Can you work these out from the model? Positions are in its coordinate system, mm. A direction names the side the tool comes from. Give positions to 0.01 mm unless a question says otherwise; leave off trailing zeros. Loops run counter-clockwise (first coordinate to the right, second up) from the corner with the lowest first, then second, coordinate; pieces in that order, holes last. Notation, with made-up numbers: (73, 67) - (81, 67) arc R32 cw to (81, 94) - close; hole circle Ø7 at (27, -12). An arc over 180 degrees is marked (long way). Answer in a Markdown table with one row per item.
from build123d import *

# Parameters (mm, degrees)
REVOLVE1_ANGLE      = 180
BOSS_EXTRUDE2_DEPTH = 8
REVOLVE2_ANGLE      = 180
SWEEP1_PROFILE_R    = 0.5
SWEEP2_PROFILE_R    = 0.5


with BuildPart() as part:
    # Sketch3 → Revolve1 (revolve)
    with BuildSketch(Plane(origin=(0, 0, 0), x_dir=(0, 0, -1), z_dir=(1, 0, 0))):
        with BuildLine():
            Line((-32, 4), (-2, 4))
            ThreePointArc((-2, 4), (-1.5, 3.5), (-1, 4))
            Line((-1, 4), (0, 4))
            Line((0, 4), (0, 0))
            Line((0, 0), (-32, 0))
            Line((-32, 0), (-32, 4))
        make_face()
    revolve(axis=Axis((0, 0, 32.603933811), (0, 0, -1)), revolution_arc=REVOLVE1_ANGLE)

    # Sketch4 → Boss-Extrude2 (add)
    with BuildSketch(Plane.ZY):
        with BuildLine():
            Line((0, 4), (0, -4))
            Line((0, -4), (1, -4))
            ThreePointArc((1, -4), (1.5, -3.5), (2, -4))
            Line((2, -4), (32, -4))
            Line((32, -4), (32, 4))
            Line((32, 4), (2, 4))
            ThreePointArc((2, 4), (1.5, 3.5), (1, 4))
            Line((1, 4), (0, 4))
        make_face()
    extrude(amount=BOSS_EXTRUDE2_DEPTH)

    # Sketch5 → Revolve2 (revolve)
    with BuildSketch(Plane.ZY.offset(8)):
        with BuildLine():
            Line((0, 0), (0, 4))
            Line((0, 4), (1, 4))
            ThreePointArc((1, 4), (1.5, 3.5), (2, 4))
            Line((2, 4), (32, 4))
            Line((32, 4), (32, 0))
            Line((32, 0), (0, 0))
        make_face()
    revolve(axis=Axis((-8, 0, -3.043909687), (0, 0, 1)), revolution_arc=REVOLVE2_ANGLE)

    # Sweep1: sweep along a path in Sketch7
    with BuildLine(Plane(origin=(1.75, 0, 0), x_dir=(0, 0, -1), z_dir=(1, 0, 0))) as sweep1_path:
        Line((0, 0), (1, 0))
        ThreePointArc((1, 0), (2.414213562, -0.585786438), (3, -2))
        Line((3, -2), (3, -7))
    # Sweep1 profile (on start of the path) → Sweep1 (sweep)
    with BuildSketch(Plane(origin=(1.75, 0, 0), x_dir=(-1, 0, 0), z_dir=(0, 0, -1))):
        Circle(SWEEP1_PROFILE_R)
    sweep(path=sweep1_path.line)

    # Sweep2: sweep along a path in Sketch14
    with BuildLine(Plane.ZY.offset(9.75)) as sweep2_path:
        Line((0, 0), (-1, 0))
        ThreePointArc((-1, 0), (-2.414213562, -0.585786438), (-3, -2))
        Line((-3, -2), (-3, -7))
    # Sweep2 profile (on start of the path) → Sweep2 (sweep)
    with BuildSketch(Plane(origin=(-9.75, 0, 0), x_dir=(0, -1, 0), z_dir=(0, 0, -1))):
        Circle(SWEEP2_PROFILE_R)
    sweep(path=sweep2_path.line)


solid = part.part
Q1. Imagine slicing it at A-A, the plane x = -5.5. Write out the boundary of the cut face in (y, z).
Checked values:
| item | result |
|---|---|
| outline | (-4, 0) - (4, 0) - (4, 1) arc R0.5 cw to (4, 2) - (4, 32) - (-4, 32) - (-4, 2) arc R0.5 cw to (-4, 1) - close |
Q2. Imagine slicing it at C-C, the plane z = 7. Write out the boundary of the cut face in (x, y).
Checked values:
| item | result |
|---|---|
| outline | (-8, -4) - (0, -4) arc R4 ccw to (0, 4) - (-8, 4) arc R4 ccw to start |
Q3. For pin 1 (4 mm diameter, centred on x = -1.5, z = 3.5, fed in from -Y); pin 2 (4 mm diameter, centred on x = -6, y = 0.5, fed in from -Z), each with a flat end and sliding along its axis, tell me the tip position at first contact or that it passes through.
Checked values:
| item | result |
|---|---|
| pin 1 | stops at y = -4 |
| pin 2 | stops at z = 0 |
Q4. On a 3-axis mill with a long thin cutter (end or side, diameter ignored), from which of +Z, -Z, +X, -X, +Y, -Y can I reach the whole of each face in a straight line? I mean faces 1 (the face through (-9.262, 0.108, -0.507)), 2 (the face through (-3.9, -3.5, 1.5)). Say none if no direction works.
Checked values:
| item | result |
|---|---|
| face 1 | none |
| face 2 | +X, -X, -Y |
Q5. If we mould it in two halves opening along X, with no side actions, what happens to faces 3 (the face through (-12, 0, 17)), 4 (the face through (2.119, -4.535, -3.338)), 5 (the face through (-4, -4, 17)), 6 (the face through (-9.262, -4.535, -3.108))? For each: released by +X, released by -X, zero draft, split by the parting line, or undercut.
Checked values:
| item | result |
|---|---|
| face 3 | released by -X |
| face 4 | undercut |
| face 5 | zero draft |
| face 6 | undercut |
Q6. Imagine slicing it at B-B, the plane z = 1.5. Write out the boundary of the cut face in (x, y), and give its area (3 significant figures).
Checked values:
| item | result |
|---|---|
| outline | (-8, -3.5) - (0, -3.5) arc R3.5 ccw to (0, 3.5) - (-8, 3.5) arc R3.5 ccw to start |
| area | 94.5 mm² |
Q7. If I drill on line 1 (Z direction, x = -5, y = -3.25); line 2 (Z direction, x = 1.75, y = -2.75); line 3 (X direction, y = 0.25, z = 20.5), over which ranges is the centre line in solid material (lowest first)? Write a range as [from, to].
Checked values:
| item | result |
|---|---|
| line 1 | z = [0, 32] |
| line 2 | z = [-3.5, -2.5], [0, 32] |
| line 3 | x = [-11.99, 3.99] |
